Source: CAD feature listing. Evaluate the final solid. Frame: model axes, mm. Face numbers are marked on the shaded views. Round coordinates to 2 decimals unless told otherwise and drop trailing zeros. Loops run counter-clockwise (first coordinate to the right, second up) from the corner with the lowest first, then second, coordinate; pieces in that order, holes last.
Item 1: Section query A-A on y = -6.5. Return loops of the section in (x, z).
Item 2: Pull-direction query (Z, two-part tool) for the marked faces 1 and 2; classes: released by +Z, released by -Z, zero draft, split by the parting line, or undercut.
Item 3: First-contact query: P1, Ø6.5, axis at x = -14, z = 9, coming from the +Y side; P2, Ø8, axis at x = 0, y = -58, coming from the +Z side; P3, Ø1.8, axis at x = -0.5, z = 2.5, coming from the -Y side; P4, Ø2.5, axis at y = -136.3, z = 6, coming from the -X side. Flat tips, straight axial feed; report the tip coordinate or a pass-through.
Item 4: Ray query, L1, parallel to X at y = -115, z = 5.25; L2, parallel to X at y = -127, z = 6.5; L3, parallel to X at y = -19.5, z = 1.75. Return the intervals inside material, ascending.
Item 5: Section query B-B on z = 2. Return loops of the section in (x, y).
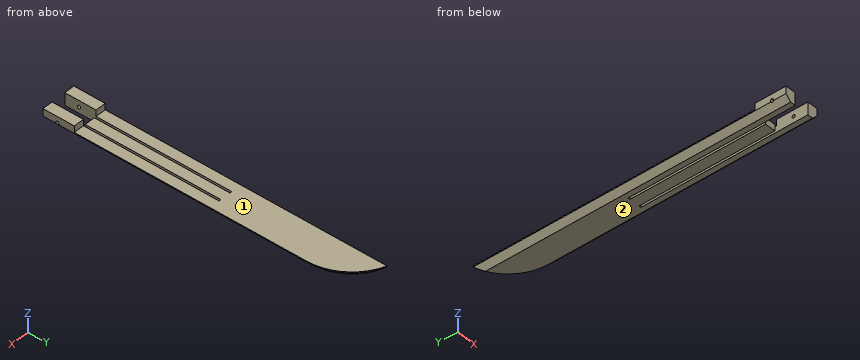
```python
from build123d import *

# Parameters (mm, degrees)
F1_DEPTH    = 6
F2_W        = 10
F2_H        = 30
F3_DEPTH    = 6
F4_R        = 1.5
F5_DEPTH    = 34.001
F6_T1_DEPTH = 242.8543856465
F7_T1_DEPTH = 325.7168298797
F7_T3_DEPTH = 265.4875378105
F7_T6_ANGLE = 86.0754516161


# Not quite as in the source:
# - a fillet or chamfer that OpenCascade refuses, or shapes differently, is made with other operations: its cross-section is extruded or revolved along the edge and cut away or added


with BuildPart() as f1:
    # F0 (on Top) → F1 (new body)
    with BuildSketch(Plane.XY):
        Polygon((7, -150), (17, -150), (17, 150), (-17, 150), (-17, -150), (-7, -150), (-7, 10), (-5, 10), (-5, -120), (5, -120), (5, 10), (7, 10), align=None)
    extrude(amount=F1_DEPTH)

    # F2 (on face) → F3 (join)
    with BuildSketch(Plane.XY.offset(6)):
        with Locations((-12, -135)):
            Rectangle(F2_W, F2_H)
        with Locations((12, -135)):
            Rectangle(F2_W, F2_H)
    extrude(amount=F3_DEPTH)

    # F4 (on face) → F5 (cut, through all)
    with BuildSketch(Plane(origin=(-17, 0, 0), x_dir=(0, -1, 0), z_dir=(-1, 0, 0))):
        with Locations((136.3040655851, 6)):
            Circle(F4_R)
    extrude(amount=-F5_DEPTH, mode=Mode.SUBTRACT)

    # F6: fillet of radius 50 on 1 edges, made by hand

    # F6_s2 → F6_t1 (cut)
    with BuildSketch(Plane.XY.offset(-118.4271928233)):
        with BuildLine():
            ThreePointArc((17, 102.6291228707), (7.6201920232, 131.7838823449), (-17, 150))
            Line((-17, 150), (17, 150))
            Line((17, 150), (17, 102.6291228707))
        make_face()
    extrude(amount=F6_T1_DEPTH, mode=Mode.SUBTRACT)

    # F7: chamfer of 5 on 3 edges, made by hand

    # F7_s2 → F7_t1 (cut)
    with BuildSketch(Plane.XZ.offset(-162.8584149398)):
        Polygon((-12, 0), (-17, 5), (-17, 0), align=None)
    extrude(amount=F7_T1_DEPTH, mode=Mode.SUBTRACT)

    # F7_s4 → F7_t3 (cut)
    with BuildSketch(Plane.XZ.offset(-102.6291228707)):
        Polygon((17, 5), (12, 0), (17, 0), align=None)
    extrude(amount=F7_T3_DEPTH, mode=Mode.SUBTRACT)

    # F7_s5 → F7_t6 (revolve, cut)
    with BuildSketch(Plane(origin=(-39.8531616504, 2.7340709455, 0), x_dir=(0, 0, 1), z_dir=(-0.9976550461, 0.0684427424, 0))):
        Polygon((0, 145.1298518112), (5, 150.1298518112), (0, 150.1298518112), align=None)
    revolve(axis=Axis((-33, 102.6291228707, 0), (0, 0, -1)), revolution_arc=F7_T6_ANGLE, mode=Mode.SUBTRACT)


solid = f1.part
```
Data:
1. outline: (-17, 5) - (-12, 0) - (-7, 0) - (-7, 6) - (-17, 6) - close; (-5, 0) - (5, 0) - (5, 6) - (-5, 6) - close; (7, 0) - (12, 0) - (17, 5) - (17, 6) - (7, 6) - close
2. face 1: released by +Z
2. face 2: released by -Z
3. P1: stops at y = 149.37
3. P2: stops at z = 6
3. P3: stops at y = -120
3. P4: passes through
4. L1: x = -17 to -7, -5 to 5, 7 to 17
4. L2: x = -17 to -7, 7 to 17
4. L3: x = -13.75 to -7, -5 to 5, 7 to 13.75
5. outline: (-14, -150) - (-7, -150) - (-7, 10) - (-5, 10) - (-5, -120) - (5, -120) - (5, 10) - (7, 10) - (7, -150) - (14, -150) - (14, 102.63) arc R47 ccw to (-14, 145.62) - close
